Work out the finished part from the listing and answer in its coordinate system (mm). Give positions to 0.01 mm unless a question says otherwise; leave off trailing zeros. Loops run counter-clockwise (first coordinate to the right, second up) from the corner with the lowest first, then second, coordinate; pieces in that order, holes last. Notation, with made-up numbers: M 85.25,5 L 109.25,5 A32 ccw 109.25,37 Z; hole C -20,-14.5 d7. An arc over 180 degrees is marked long. Answer as a JSON object with one key per item and string values. Group by question number.
```python
from build123d import *

# Parameters (mm, degrees)
SKETCH_W        = 185
SKETCH_H        = 145
PAD_DEPTH       = 3.7
SKETCH001_W     = 48.165349
SKETCH001_H     = 70
POCKET_DEPTH    = 5
POCKET001_DEPTH = 5


with BuildPart() as part:
    # Sketch → Pad (new body)
    with BuildSketch(Plane.XY):
        Rectangle(SKETCH_W, SKETCH_H)
    extrude(amount=PAD_DEPTH)

    # Sketch001 (on Face6 of Pad) → Pocket (cut)
    with BuildSketch(Plane.XY.offset(3.7)):
        with Locations((-18.417326, 17.5)):
            Rectangle(SKETCH001_W, SKETCH001_H)
    extrude(amount=-POCKET_DEPTH, mode=Mode.SUBTRACT)

    # Sketch003 (on Face5 of Pocket) → Pocket001 (cut)
    with BuildSketch(Plane.XY.offset(3.7)):
        with BuildLine():
            ThreePointArc((-21.417326, 62.5), (-23.917326, 60), (-21.417326, 57.5))
            Line((-21.417326, 57.5), (-15.417326, 57.5))
            ThreePointArc((-15.417326, 57.5), (-12.917326, 60), (-15.417326, 62.5))
            Line((-21.417326, 62.5), (-15.417326, 62.5))
        make_face()
        with BuildLine():
            Line((-21.416062, -22.5), (-15.418589, -22.5))
            ThreePointArc((-15.418589, -27.5), (-12.918589, -25), (-15.418589, -22.5))
            Line((-21.416062, -27.5), (-15.418589, -27.5))
            ThreePointArc((-21.416062, -22.5), (-23.916062, -25), (-21.416062, -27.5))
        make_face()
        with BuildLine():
            ThreePointArc((-47.5, 42.5), (-50, 45), (-52.5, 42.5))
            Line((-52.5, 42.5), (-52.5, 36.5))
            ThreePointArc((-52.5, 36.5), (-50, 34), (-47.5, 36.5))
            Line((-47.5, 42.5), (-47.5, 36.5))
        make_face()
        with BuildLine():
            ThreePointArc((15.665349, 42.5), (13.165349, 45), (10.665349, 42.5))
            Line((10.665349, 42.5), (10.665349, 36.5))
            ThreePointArc((10.665349, 36.5), (13.165349, 34), (15.665349, 36.5))
            Line((15.665349, 42.5), (15.665349, 36.5))
        make_face()
        with BuildLine():
            ThreePointArc((-47.5, -1.5), (-50, 1), (-52.5, -1.5))
            Line((-52.5, -1.5), (-52.5, -7.5))
            ThreePointArc((-52.5, -7.5), (-50, -10), (-47.5, -7.5))
            Line((-47.5, -1.5), (-47.5, -7.5))
        make_face()
        with BuildLine():
            ThreePointArc((15.665349, -1.5), (13.165349, 1), (10.665349, -1.5))
            Line((10.665349, -1.5), (10.665349, -7.5))
            ThreePointArc((10.665349, -7.5), (13.165349, -10), (15.665349, -7.5))
            Line((15.665349, -1.5), (15.665349, -7.5))
        make_face()
    extrude(amount=-POCKET001_DEPTH, mode=Mode.SUBTRACT)


solid = part.part
```
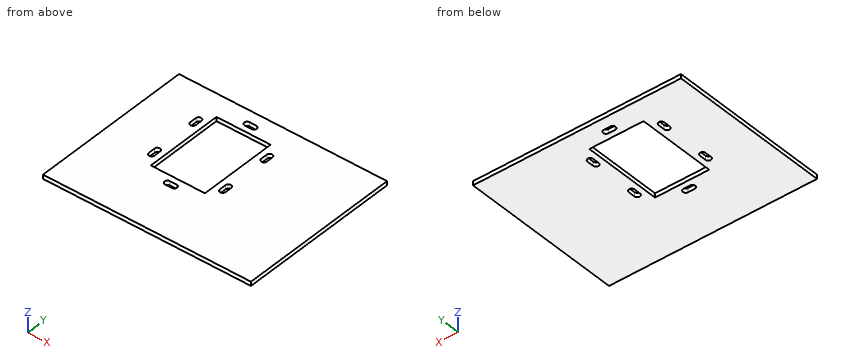
Item 1: Find the intervals of material crossed by probe 1 along X at (y, z) = (-7.5, 1.05); probe 2 along Y at (x, z) = (-31, 2.7); probe 3 along X at (y, z) = (7, 2.7), in increasing order. Write a range as [from, to].
Item 2: A cutting plane is placed at D-D (z = 1.4). Give the number of separate pieces and of enclosed holes in the cut face, and give its area (3 significant figures).
Item 3: A cutting plane is placed at C-C (x = -50). Determine the outline of the cut face in (y, z), and give its area (3 significant figures).
Item 4: A cutting plane is placed at A-A (y = -25). Determine the outline of the cut face in (x, z).
Item 5: A cutting plane is placed at B-B (x = -26.5). Determine the outline of the cut face in (y, z), and give its area (4 significant figures).
The answers:
{
 "1": {"probe 1": "x = [-92.5, -52.5], [-47.5, -42.5], [5.67, 10.67], [15.67, 92.5]", "probe 2": "y = [-72.5, -17.5], [52.5, 72.5]", "probe 3": "x = [-92.5, -42.5], [5.67, 92.5]"},
 "2": {"separate pieces": "1", "enclosed holes": "7", "area": "23,200 mm^2"},
 "3": {"outline": "M -72.5,0 L -10,0 L -10,3.7 L -72.5,3.7 Z; M 1,0 L 34,0 L 34,3.7 L 1,3.7 Z; M 45,0 L 72.5,0 L 72.5,3.7 L 45,3.7 Z", "area": "455 mm^2"},
 "4": {"outline": "M -92.5,0 L -23.92,0 L -23.92,3.7 L -92.5,3.7 Z; M -12.92,0 L 92.5,0 L 92.5,3.7 L -12.92,3.7 Z"},
 "5": {"outline": "M -72.5,0 L -17.5,0 L -17.5,3.7 L -72.5,3.7 Z; M 52.5,0 L 72.5,0 L 72.5,3.7 L 52.5,3.7 Z", "area": "277.5 mm^2"}
}
